```python
from build123d import *

# Parameters (mm, degrees)
EXTRUDE_1_DEPTH = 3


with BuildPart() as part:
    # 草图1 → 旋转1 (revolve)
    with BuildSketch(Plane.XY, mode=Mode.PRIVATE) as revolve_1_sk:
        Polygon((0, 70), (0, 0), (10, 10), (10, 63), (3, 63), (3, 70), align=None)
    revolve(revolve_1_sk.sketch.rotate(Axis((0, 70, 0), (0, -1, 0)), 180), axis=Axis((0, 70, 0), (0, -1, 0)))

    # 草图2 → 凸台-拉伸1 (add, symmetric)
    with BuildSketch(Plane.XY):
        Polygon((-14, 72), (-7.07179677, 68), (-7.07179677, 70), (13, 70), (13, 74), (-7.07179677, 74), (-7.07179677, 76), align=None)
    extrude(amount=EXTRUDE_1_DEPTH, both=True)


solid = part.part
```
Read the model definition and answer for the solid it produces. Units are mm, in the model's axes. A direction names the side the tool comes from. Round coordinates to 2 decimals unless told otherwise and drop trailing zeros. Write each loop counter-clockwise with the first axis right and the second up, starting at its lowest first coordinate (ties: lowest second). Pieces come first, ordered by that corner, then holes. Notation, with made-up numbers: (-5.75, -34.75) -> (19.25, -34.75) arc R20 cw to (19.25, -3.75) -> close; hole circle Ø4 at (89, -5.5). An arc over 180 degrees is marked (long way). Answer in a Markdown table with one row per item. Add a question column.
1) Given P1, Ø5, axis at x = 4, z = -0.5, coming from the -Y side; P2, Ø1.8, axis at x = -5, z = 0, coming from the -Y side; P3, Ø5, axis at x = 3, z = 1, coming from the +Y side, each flat-ended and moving along its own axis, determine where each tip first touches the part or whether it passes through.
2) Consider line 1 (Z direction, x = 4.5, y = 73); line 2 (Y direction, x = -3.5, z = 1.5); line 3 (Z direction, x = 7.75, y = 30.5). Determine where each line is inside the solid, lowest interval first.
3) Find section A-A, the plane y = 13. Determine the outline of the cut face in (x, z).
4) Which of the six approach directions +Z, -Z, +X, -X, +Y, -Y give full straight-line access (tool end or side, diameter ignored) to faces 4 (the face through (-7.072, 69, 0)), 5 (the face through (-1, 72, 3)), 6 (the face through (3, 74, 0))?
5) Determine the mould class of faces 1 (the face through (-1, 72, -3)), 2 (the face through (-2.86, 66.55, -0.9)), 3 (the face through (-10.487, 74.028, 0.042)) for opening direction Y: pulls with the +Y half, pulls with the -Y half, needs draft (parallel to the pull), parting line crosses it, or undercut.
Findings below:
| question | item | result |
|---|---|---|
| 1 | P1 | y = 1.53 |
| 1 | P2 | y = 4.1 |
| 1 | P3 | y = 74 |
| 2 | line 1 | -3 to 3 |
| 2 | line 2 | 3.81 to 63, 70 to 74 |
| 2 | line 3 | -6.32 to 6.32 |
| 3 | outline | circle Ø20 at (0, 0) |
| 4 | face 4 | +Z, -Z |
| 4 | face 5 | +Z, +X, -X, +Y |
| 4 | face 6 | +Z, -Z, +X, +Y |
| 5 | face 1 | needs draft |
| 5 | face 2 | undercut |
| 5 | face 3 | pulls with the +Y half |
